For this review, take the finished solid that the model builds, in its own axes (mm). A direction names the side the tool comes from. Round coordinates to 2 decimals unless told otherwise and drop trailing zeros. Loops run counter-clockwise (first coordinate to the right, second up) from the corner with the lowest first, then second, coordinate; pieces in that order, holes last.
```python
from build123d import *

# Parameters (mm, degrees)
SKETCH1_W               = 254
SKETCH1_H               = 127
BOSS_EXTRUDE1_DEPTH     = 6.35
SKETCH2_W               = 18.796
SKETCH2_H               = 6.35
CUT_EXTRUDE1_DEPTH      = 7.35
CUT_EXTRUDE1_DEPTH_BACK = 6.35
SKETCH3_W               = 12.876244412
SKETCH3_H               = 6.459801397
SKETCH3_W_2             = 12.7
SKETCH3_H_2             = 6.35
CUT_EXTRUDE3_DEPTH      = 127
CUT_EXTRUDE3_DEPTH_BACK = 127
SKETCH4_W               = 12.876244412
SKETCH4_H               = 6.459801397
CUT_EXTRUDE4_DEPTH      = 127
CUT_EXTRUDE4_DEPTH_BACK = 127


with BuildPart() as part:
    # Sketch1 → Boss-Extrude1 (new body)
    with BuildSketch(Plane(origin=(0, 0, 0), x_dir=(1, 0, 0), z_dir=(0, 1, 0))):
        Rectangle(SKETCH1_W, SKETCH1_H)
    extrude(amount=BOSS_EXTRUDE1_DEPTH)

    # Sketch2 → Cut-Extrude1 (cut, two sides)
    with BuildSketch(Plane(origin=(0, 0, 0), x_dir=(1, 0, 0), z_dir=(0, 1, 0))) as cut_extrude1_sk:
        Polygon((-107.95, -63.5), (-107.95, -57.15), (-120.65, -57.15), (-120.65, -50.8), (-127, -50.8), (-127, -63.5), align=None)
        with Locations((0, -60.325)):
            Rectangle(SKETCH2_W, SKETCH2_H)
        Polygon((-127, 50.8), (-120.65, 50.8), (-120.65, 57.15), (-107.95, 57.15), (-107.95, 63.5), (-127, 63.5), align=None)
        with Locations((0, 60.325)):
            Rectangle(SKETCH2_W, SKETCH2_H)
        Polygon((107.95, -63.5), (107.95, -57.15), (120.65, -57.15), (120.65, -50.8), (127, -50.8), (127, -63.5), align=None)
        Polygon((127, 50.8), (120.65, 50.8), (120.65, 57.15), (107.95, 57.15), (107.95, 63.5), (127, 63.5), align=None)
    extrude(amount=CUT_EXTRUDE1_DEPTH, mode=Mode.SUBTRACT)
    extrude(cut_extrude1_sk.sketch, amount=-CUT_EXTRUDE1_DEPTH_BACK, mode=Mode.SUBTRACT)

    # Sketch3 → Cut-Extrude3 (cut, two sides)
    with BuildSketch(Plane(origin=(0, 0, 0), x_dir=(1, 0, 0), z_dir=(0, 1, 0))) as cut_extrude3_sk:
        with Locations((-114.211877794, -53.920099302)):
            Rectangle(SKETCH3_W, SKETCH3_H)
        with Locations((-114.3, 53.975)):
            Rectangle(SKETCH3_W_2, SKETCH3_H_2)
        with Locations((114.3, -53.920099302)):
            Rectangle(SKETCH3_W_2, SKETCH3_H)
    extrude(amount=CUT_EXTRUDE3_DEPTH, mode=Mode.SUBTRACT)
    extrude(cut_extrude3_sk.sketch, amount=-CUT_EXTRUDE3_DEPTH_BACK, mode=Mode.SUBTRACT)

    # Sketch4 → Cut-Extrude4 (cut, two sides)
    with BuildSketch(Plane(origin=(0, 0, 0), x_dir=(-1, 0, 0), z_dir=(0, -1, 0))) as cut_extrude4_sk:
        with Locations((-114.211877794, 53.920099302)):
            Rectangle(SKETCH4_W, SKETCH4_H)
    extrude(amount=CUT_EXTRUDE4_DEPTH, mode=Mode.SUBTRACT)
    extrude(cut_extrude4_sk.sketch, amount=-CUT_EXTRUDE4_DEPTH_BACK, mode=Mode.SUBTRACT)


solid = part.part
```
(1) The part is to be moulded in two halves that separate along X. For faces 1 (the flat face through (107.95, 3, -60)), 2 (the flat face through (9.398, 3, 60)), 3 (the flat face through (58, 3, 63.5)), say which applies: pulls with the +X half, pulls with the -X half, needs draft (parallel to the pull), parting line crosses it, or undercut.
(2) For L1, parallel to X at y = 5.5, z = -54.5; L2, parallel to X at y = 0.5, z = 56.5, list the stretches that pass through material, from the lowest coordinate up.
(3) Insertion check: pin 1 Ø1.9 at (y, z) = (2, -59) entering from +X; pin 2 Ø3 at (x, y) = (122.5, 4.5) entering from +Z; pin 3 Ø3 at (y, z) = (4, 61.5) entering from -X. Each pin has a flat end and moves straight along its axis. Give the tip position at first contact, or say it passes through.
(4) Add section B-B (x = -5). Give the boundary of the cut face in (y, z), plus the area to 3 significant figures.
(5) Add section C-C (z = -53.5). Give the boundary of the cut face in (x, y), plus the area to 3 significant figures.
(6) For faces 4 (the flat face through (-118, 3, -50.8)), 5 (the flat face through (-124, 3, 50.8)), 6 (the flat face through (0, 3, -57.15)), 7 (the flat face through (124, 3, -50.8)), list the 3-axis set-ups (+Z, -Z, +X, -X, +Y, -Y) from which the entire face can be reached by the end or side of a thin tool; tool diameter is ignored.
Outcome:
1. face 1: pulls with the +X half
1. face 2: undercut
1. face 3: needs draft
2. L1: x = -107.95 to 107.77
2. L2: x = -107.77 to 107.95
3. pin 1: stops at x = 107.95
3. pin 2: stops at z = 50.8
3. pin 3: stops at x = -107.95
4. outline: (0, -57.15) - (6.35, -57.15) - (6.35, 57.15) - (0, 57.15) - close
4. area: 726 mm2
5. outline: (-107.95, 0) - (107.77, 0) - (107.77, 6.35) - (-107.95, 6.35) - close
5. area: 1,370 mm2
6. face 4: -Z, -X, +Y, -Y
6. face 5: +Z, -X, +Y, -Y
6. face 6: -Z, +Y, -Y
6. face 7: -Z, +X, +Y, -Y
